```python
from build123d import *

# Parameters (mm, degrees)
BOSS_EXTRUDE1_DEPTH   = 228.6
SKETCH3_R             = 4.7625
CUT_EXTRUDE1_DEPTH    = 229.6
F_4_40_TAPPED_HOLE1_D = 2.2606
CUT_EXTRUDE2_DEPTH    = 229.6
SKETCH7_W             = 48.175
SKETCH7_H             = 138.175
CUT_EXTRUDE3_DEPTH    = 12.7
SKETCH8_W             = 48.175
SKETCH8_H             = 138.175
CUT_EXTRUDE4_DEPTH    = 12.7


with BuildPart() as part:
    # Sketch1 → Boss-Extrude1 (new body)
    with BuildSketch(Plane(origin=(0, 0, 0), x_dir=(1, 0, 0), z_dir=(0, 1, 0))):
        with BuildLine():
            Line((-65.349491008, -9.525), (65.349491008, -9.525))
            ThreePointArc((65.349491008, -9.525), (66.04, 0), (65.349491008, 9.525))
            Line((65.349491008, 9.525), (-65.349491008, 9.525))
            ThreePointArc((-65.349491008, 9.525), (-66.04, 0), (-65.349491008, -9.525))
        make_face()
    extrude(amount=-BOSS_EXTRUDE1_DEPTH)

    # Sketch3 → Cut-Extrude1 (cut, through all)
    with BuildSketch(Plane(origin=(0, 0, 0), x_dir=(1, 0, 0), z_dir=(0, 1, 0))):
        Circle(SKETCH3_R)
    extrude(amount=-CUT_EXTRUDE1_DEPTH, mode=Mode.SUBTRACT)

    # #4-40 Tapped Hole1 (through all)
    with Locations(Plane.XY.offset(9.525)):
        with Locations((-50.895394878, -56.7192), (-12.604605122, -56.7192), (-12.604605122, -214.6808), (-50.895394878, -214.6808), (12.604605122, -56.7192), (50.895394878, -56.7192), (12.604605122, -214.6808), (50.895394878, -214.6808)):
            Hole(F_4_40_TAPPED_HOLE1_D / 2)

    # Sketch6 → Cut-Extrude2 (cut, through all)
    with BuildSketch(Plane.XZ.offset(228.6)):
        with BuildLine():
            Line((59.613633731, 3.175), (65.963633731, 3.175))
            ThreePointArc((65.963633731, 3.175), (66.04, 0), (65.963633731, -3.175))
            Line((65.963633731, -3.175), (59.613633731, -3.175))
            Line((59.613633731, -3.175), (59.613633731, 3.175))
        make_face()
    extrude(amount=-CUT_EXTRUDE2_DEPTH, mode=Mode.SUBTRACT)

    # Sketch7 → Cut-Extrude3 (cut)
    with BuildSketch(Plane.XY.offset(9.525)):
        with Locations((-31.75, -135.7)):
            Rectangle(SKETCH7_W, SKETCH7_H)
    extrude(amount=-CUT_EXTRUDE3_DEPTH, mode=Mode.SUBTRACT)

    # Sketch8 → Cut-Extrude4 (cut)
    with BuildSketch(Plane(origin=(0, 0, -9.525), x_dir=(-1, 0, 0), z_dir=(0, 0, -1))):
        with Locations((-31.75, -135.7)):
            Rectangle(SKETCH8_W, SKETCH8_H)
    extrude(amount=-CUT_EXTRUDE4_DEPTH, mode=Mode.SUBTRACT)


solid = part.part
```
The listing builds one solid part. Answer for the finished solid, in the listing's coordinates (mm). A direction names the side the tool comes from. Coordinates: 2 decimals unless noted, no trailing zeros. Write each loop counter-clockwise with the first axis right and the second up, starting at its lowest first coordinate (ties: lowest second). Pieces come first, ordered by that corner, then holes. Notation, with made-up numbers: (88, 35.5) -> (111, 35.5) arc R6 cw to (111, 41.5) -> close; hole circle Ø9 at (0, 29). An arc over 180 degrees is marked (long way). Write each question's results on one line, items separated by ' | '. Start each with the question number.
1) A cutting plane is placed at B-B (z = 0). Count the separate pieces of the cut face and the enclosed holes in it, then the cut area to 3 significant figures.
2) A cutting plane is placed at C-C (y = -121). Determine the outline of the cut face in (x, z) (1 decimal), then the cut area to 3 significant figures.
3) A cutting plane is placed at A-A (x = 0). Determine the outline of the cut face in (y, z) (1 decimal), then the cut area to 3 significant figures.
4) A tool of negligible diameter and unlimited length cuts with its end or side. For faces 4 (the flat face through (63, -116, -3.175)), 5 (the flat face through (-55.838, -137, 3)), 6 (the flat face through (-1, -228.6, -6)), 7 (the flat face through (32, -66.612, -3)), 8 (the flat face through (1, -113, -9.525)), from which of +Z, -Z, +X, -X, +Y, -Y can it reach the whole face along a straight path? Write none if from no direction.
5) A cutting plane is placed at D-D (x = 28.5). Determine the outline of the cut face in (y, z) (1 decimal), then the cut area to 3 significant figures.
6) Flat-ended cylindrical pins translate along their axes: pin 1 Ø2 at (y, z) = (-45, -1.5) entering from +X; pin 2 Ø3 at (x, y) = (-12.6, -56.72) entering from -Z (3 decimals); pin 3 Ø1.4 at (x, y) = (50.9, -214.68) entering from -Z; pin 4 Ø3 at (y, z) = (-108.5, 5) entering from -X. Find the tip coordinate at first contact, or state that the pin passes through.
7) Straight lines are drawn through the part: probe 1 along X at (y, z) = (-169, 0.25); probe 2 along Y at (x, z) = (-50.5, 5.75); probe 3 along X at (y, z) = (-104, -3). For each, find the intervals that lie inside material, in ascending order.
8) For a pull along Y with two mould halves and no side action, classify faces 1 (the flat face through (32, -135, 3.175)), 2 (the flat face through (59.614, -116, 0)), 3 (the flat face through (-1, 0, -6)) as +Y half, -Y half, draft (parallel to the pull), parting line (faces both ways), or undercut.
Values follow:
1) separate pieces: 2 | enclosed holes: 10 | area: 13,200 mm²
2) outline: (-65.3, -9.5) -> (7.7, -9.5) -> (7.7, 3.2) -> (55.8, 3.2) -> (55.8, -9.5) -> (65.3, -9.5) arc R66 ccw to (66, -3.2) -> (59.6, -3.2) -> (59.6, 3.2) -> (66, 3.2) arc R66 ccw to (65.3, 9.5) -> (-7.7, 9.5) -> (-7.7, -3.2) -> (-55.8, -3.2) -> (-55.8, 9.5) -> (-65.3, 9.5) arc R66 ccw to start; hole circle Ø9.5 at (0, 0) | area: 1,170 mm²
3) outline: (-228.6, -9.5) -> (0, -9.5) -> (0, -4.8) -> (-228.6, -4.8) -> close; (-228.6, 4.8) -> (0, 4.8) -> (0, 9.5) -> (-228.6, 9.5) -> close | area: 2,180 mm²
4) face 4: +X, +Y, -Y | face 5: +Z | face 6: +Z, -Z, +X, -X, -Y | face 7: -Z | face 8: -Z, +X, -X, +Y, -Y
5) outline: (-228.6, -9.5) -> (-204.8, -9.5) -> (-204.8, 3.2) -> (-66.6, 3.2) -> (-66.6, -9.5) -> (0, -9.5) -> (0, 9.5) -> (-228.6, 9.5) -> close | area: 2,600 mm²
6) pin 1: x = 59.61 | pin 2: z = -9.525 | pin 3: through | pin 4: x = -65.95
7) probe 1: -66.04 to -55.84, -7.66 to -4.76, 4.76 to 7.66, 55.84 to 59.61 | probe 2: -228.6 to -215.74, -213.62 to -204.79, -66.61 to -57.78, -55.66 to 0 | probe 3: -65.97 to -55.84, -7.66 to -3.7, 3.7 to 7.66, 55.84 to 59.61
8) face 1: undercut | face 2: draft | face 3: +Y half
